```python
from build123d import *

# Parameters (mm, degrees)
SKETCH1_W           = 20.4
SKETCH1_H           = 20.4
SKETCH1_W_2         = 16.4
SKETCH1_H_2         = 16.4
BOSS_EXTRUDE1_DEPTH = 50
SKETCH2_W           = 20.4
SKETCH2_H           = 20.4
SKETCH2_W_2         = 13.834702386
SKETCH2_H_2         = 14.497254018
BOSS_EXTRUDE2_DEPTH = 3
SKETCH3_R           = 1
SKETCH3_R_2         = 1.5
CUT_EXTRUDE1_DEPTH  = 55.956346312
FILLET1_R           = 1


with BuildPart() as part:
    # Sketch1 → Boss-Extrude1 (new body)
    with BuildSketch(Plane.XY):
        Rectangle(SKETCH1_W, SKETCH1_H)
        Rectangle(SKETCH1_W_2, SKETCH1_H_2, mode=Mode.SUBTRACT)
    extrude(amount=-BOSS_EXTRUDE1_DEPTH)

    # Sketch2 → Boss-Extrude2 (add)
    with BuildSketch(Plane.XY):
        Rectangle(SKETCH2_W, SKETCH2_H)
        Rectangle(SKETCH2_W_2, SKETCH2_H_2, mode=Mode.SUBTRACT)
    extrude(amount=BOSS_EXTRUDE2_DEPTH)

    # Sketch3 → Cut-Extrude1 (cut, through all)
    with BuildSketch(Plane(origin=(10.2, 0, 0), x_dir=(0, 0, -1), z_dir=(1, 0, 0))):
        with Locations((20.5, 0)):
            Circle(SKETCH3_R)
        with Locations((9.5, 0)):
            Circle(SKETCH3_R_2)
        with Locations((33.5, 0)):
            Circle(SKETCH3_R)
        with Locations((44.5, 0)):
            Circle(SKETCH3_R_2)
    extrude(amount=-CUT_EXTRUDE1_DEPTH, mode=Mode.SUBTRACT)

    # Fillet1
    fillet1_edges = [part.edges().sort_by_distance(p)[0] for p in [
        (8.2, 0, -50),
        (0, -8.2, -50),
        (-8.2, 0, -50),
        (0, 8.2, -50),
    ]]
    fillet(fillet1_edges, radius=FILLET1_R)


solid = part.part
```
Could you check a few things on this model? Use its own coordinates, in mm. A direction names the side the tool comes from. Coordinates: 2 decimals unless noted, no trailing zeros. Order: outer loops, then holes, each group sorted by start corner. A loop starts at its lowest first (then second) coordinate and runs counter-clockwise, first axis right, second up. Notation, with made-up numbers: M -19,50.5 L -1,50.5 A27 cw -1,86.5 Z; hole C 78,14 d3. An arc over 180 degrees is marked long. Use one line per item in the form item = value. Start each with the question number.
1. Suppose I cut it at C-C on z = -32. Write out the boundary of the cut face in (x, y).
2. Suppose I cut it at D-D on y = 0. Count the separate pieces of the cut face and the enclosed holes in it, then the cut area to 3 significant figures.
3. For pin 1 (3 mm diameter, centred on x = 1, y = 4.5, fed in from -Z), with a flat end and sliding along its axis, tell me the tip position at first contact or that it passes through.
4. We'd pull the mould along Y, two halves only. Please class faces 1 (the flat face through (0, -10.2, -24)), 2 (the flat face through (8.2, 0, -24)), 3 (the cylindrical face through (-9.2, 0, -19.5)), 4 (the flat face through (-10.2, 0, -24)): +Y half, -Y half, draft (parallel to the pull), parting line (faces both ways), or undercut.
5. On a 3-axis mill with a long thin cutter (end or side, diameter ignored), from which of +Z, -Z, +X, -X, +Y, -Y can I reach the whole of each face in a straight line? I mean faces 5 (the flat face through (-9, 0, 3)), 6 (the flat face through (0, -7.249, 1)), 7 (the cylindrical face through (8.501, 0.129, -49.715)). Say none if no direction works.
6. Suppose I cut it at B-B on x = 2.75. Write out the boundary of the cut face in (y, z), then the cut area to 3 significant figures.
7. Please list where these lines run through material, in increasing order: line 1 (X direction, y = 2.75, z = -32.5); line 2 (Y direction, x = 9.45, z = -20.5).
8. Suppose I cut it at A-A on z = -9.5. Write out the boundary of the cut face in (x, y).
Geometry says:
q1.outline = M -10.2,-10.2 L 10.2,-10.2 L 10.2,10.2 L -10.2,10.2 Z; hole M -8.2,-8.2 L 8.2,-8.2 L 8.2,8.2 L -8.2,8.2 Z
q2.separate_pieces = 10
q2.enclosed_holes = 0
q2.area = 179 mm^2
q3.pin_1 = through
q4.face_1 = -Y half
q4.face_2 = undercut
q4.face_3 = undercut
q4.face_4 = draft
q5.face_5 = +Z, +X, -X, +Y, -Y
q5.face_6 = +Z, -Z
q5.face_7 = -Z
q6.outline = M -10.2,-50 L -9.2,-50 A1 ccw -8.2,-49 L -8.2,0 L -7.25,0 L -7.25,3 L -10.2,3 Z; M 7.25,0 L 8.2,0 L 8.2,-49 A1 ccw 9.2,-50 L 10.2,-50 L 10.2,3 L 7.25,3 Z
q6.area = 217 mm^2
q7.line_1 = -10.2 to -8.2, 8.2 to 10.2
q7.line_2 = -10.2 to -1, 1 to 10.2
q8.outline = M -10.2,-10.2 L 10.2,-10.2 L 10.2,-1.5 L 8.2,-1.5 L 8.2,-8.2 L -8.2,-8.2 L -8.2,-1.5 L -10.2,-1.5 Z; M -10.2,1.5 L -8.2,1.5 L -8.2,8.2 L 8.2,8.2 L 8.2,1.5 L 10.2,1.5 L 10.2,10.2 L -10.2,10.2 Z
